```python
from build123d import *

# Parameters (mm, degrees)
SKETCH3_R          = 2.5
CUT_EXTRUDE1_DEPTH = 10


with BuildPart() as part:
    # Sketch1 → Revolve1 (revolve)
    with BuildSketch(Plane(origin=(0, 0, 0), x_dir=(1, 0, 0), z_dir=(0, 1, 0))):
        Polygon((0, 11), (-7.2, 11), (-7.2, 9.2), (-30, 9.2), (-30, 0), (-18, 0), (-18, 4), (0, 4), (5, 4), (5, 14), (0, 14), align=None)
    revolve(axis=Axis((-18, 0, 0), (-1, 0, 0)))

    # Sketch3 → Cut-Extrude1 (cut)
    with BuildSketch(Plane(origin=(0, 0, 0), x_dir=(1, 0, 0), z_dir=(0, 1, 0))):
        with Locations((-11, 0)):
            Circle(SKETCH3_R)
    extrude(amount=-CUT_EXTRUDE1_DEPTH, mode=Mode.SUBTRACT)


solid = part.part
```
The model under review builds one solid part; all positions refer to its coordinate system, in mm. A direction names the side the tool comes from. Give positions to 0.01 mm unless a question says otherwise; leave off trailing zeros. Write each loop counter-clockwise with the first axis right and the second up, starting at its lowest first coordinate (ties: lowest second). Pieces come first, ordered by that corner, then holes. Notation, with made-up numbers: M 88.25,84 L 141.25,84 A6 cw 141.25,91 Z; hole C -12,43 d8. An arc over 180 degrees is marked long. Write item = value, one per line. Start each with the question number.
Q1. We need section A-A (z = 0). State the section outline as (x, y) points, plus the area to 3 significant figures.
Q2. We need section D-D (z = -10). State the section outline as (x, y) points, plus the area to 3 significant figures.
Q3. Mouldability with a two-part tool opening along Y and no side actions: class faces 4 (the face through (-6.339, 3.905, 0.867)), 5 (the face through (-18, 0, 0)), 6 (the face through (2.465, 5.362, -12.932)), 7 (the face through (5, 3, 3)) as released by +Y, released by -Y, zero draft, split by the parting line, or undercut.
Q4. Machinability: for faces 1 (the face through (-18.76, 8.981, 1.994)), 2 (the face through (-8.615, -6.123, -0.751)), 3 (the face through (-30, 0, 0)), which of the approach directions +Z, -Z, +X, -X, +Y, -Y give a long, thin tool a straight path to every point of the face, cutting with its end or side? Answer none if there is none.
Q5. We need section C-C (x = -4.5). State the section outline as (y, z) points, plus the area to 3 significant figures.
Q6. We need section B-B (y = 0). State the section outline as (x, z) points.
Q7. Clearance check with flat-ended pins moving along their axes: pin 1 (1.5 mm diameter, centred on x = -9, z = 2, fed in from +Y); pin 2 (10 mm diameter, centred on x = -21.5, y = 8, fed in from -Z); pin 3 (2 mm diameter, centred on x = -15.5, z = 8.5, fed in from +Y). State where each tip first meets the part, or that it passes through.
Q8. For line 1 (X direction, y = -8, z = 0); line 2 (Z direction, x = -3.25, y = 0); line 3 (Y direction, x = -11.5, z = 0), list the stretches that pass through material, from the lowest coordinate up.
Result set:
q1.outline = M -30,-9.2 L -13.5,-9.2 L -13.5,-4 L -18,-4 L -18,4 L 5,4 L 5,14 L 0,14 L 0,11 L -7.2,11 L -7.2,9.2 L -30,9.2 Z; M -8.5,-9.2 L -7.2,-9.2 L -7.2,-11 L 0,-11 L 0,-14 L 5,-14 L 5,-4 L -8.5,-4 Z
q1.area = 508 mm2
q2.outline = M -7.2,-4.58 L 0,-4.58 L 0,-9.8 L 5,-9.8 L 5,9.8 L 0,9.8 L 0,4.58 L -7.2,4.58 Z
q2.area = 164 mm2
q3.face_4 = undercut
q3.face_5 = undercut
q3.face_6 = split by the parting line
q3.face_7 = zero draft
q4.face_1 = -X
q4.face_2 = -Y
q4.face_3 = +Z, -Z, -X, +Y, -Y
q5.outline = C 0,0 d22; hole C 0,0 d8
q5.area = 330 mm2
q6.outline = M -30,-9.2 L -7.2,-9.2 L -7.2,-11 L 0,-11 L 0,-14 L 5,-14 L 5,-4 L -18,-4 L -18,4 L 5,4 L 5,14 L 0,14 L 0,11 L -7.2,11 L -7.2,9.2 L -30,9.2 Z
q7.pin_1 = 9.11
q7.pin_2 = -8.7
q7.pin_3 = 5.33
q8.line_1 = -30 to -13.5, -8.5 to 5
q8.line_2 = -11 to -4, 4 to 11
q8.line_3 = 4 to 9.2
